Source: three-view drawing plus pictorial views. Frame: mm from the lowest corner of the part. A direction names the side the tool comes from. Give positions to 0.01 mm unless a question says otherwise; leave off trailing zeros. Loops run counter-clockwise (first coordinate to the right, second up) from the corner with the lowest first, then second, coordinate; pieces in that order, holes last. Notation, with made-up numbers: (-37, -9) -> (-24, -9) arc R37 cw to (-24, 29) -> close; hole circle Ø2 at (16, 61). An arc over 180 degrees is marked (long way). Answer as a JSON object with one key per item and string values. Group by question number.
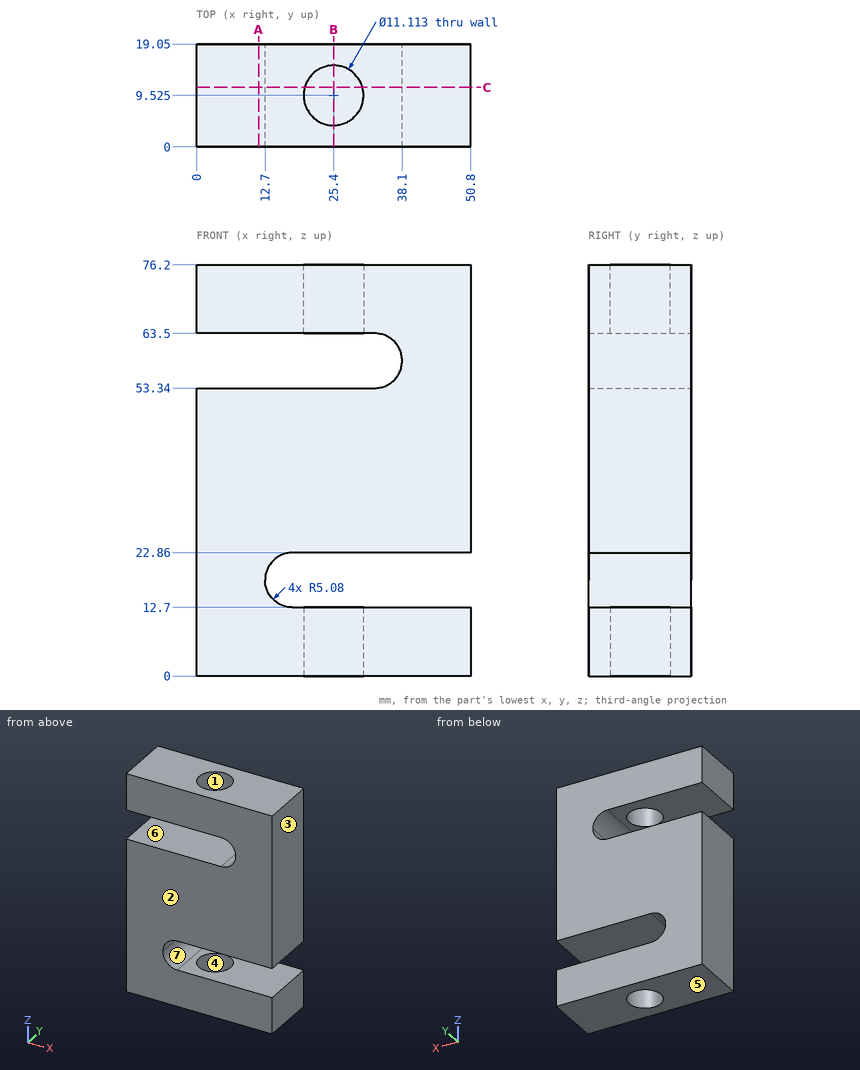
(1) Section query B-B on x = 25.4. Return the cut outline in (y, z).
(2) Section query C-C on y = 11. State how many separate pieces and enclosed holes the cut face has, plus the area to 3 significant figures.
(3) Access query for the marked faces 4, 5, 6 and 7. Directions: +Z, -Z, +X, -X, +Y, -Y. A direction counts if a zero-diameter tool reaches every point of the face in a straight line with its end or side. Return the directions, or none.
(4) First-contact query: pin 1 (6 mm diameter, centred on x = 24, y = 4.5, fed in from -Z); pin 2 (9 mm diameter, centred on x = 25.4, y = 9.525, fed in from -Z); pin 3 (4 mm diameter, centred on y = 5, z = 18, fed in from +X). Flat tips, straight axial feed; report the tip coordinate or a pass-through.
(5) Mould query, pull axis X, two halves, no side actions, for the marked faces 1, 2 and 3. Classes: pulls with the +X half, pulls with the -X half, needs draft (parallel to the pull), parting line crosses it, or undercut.
(6) Section query A-A on x = 11.5. Return the cut outline in (y, z), plus the area to 3 significant figures.
(7) Material intervals for line 1 (Z direction, x = 30.5, y = 2.5); line 2 (Y direction, x = 25.4, z = 67); line 3 (Z direction, x = 46.5, y = 2.75), sorted ascending. Write a range as from..to.
Result:
{
 "1": {"outline": "(0, 0) -> (3.97, 0) -> (3.97, 12.7) -> (0, 12.7) -> close; (0, 22.86) -> (19.05, 22.86) -> (19.05, 53.34) -> (0, 53.34) -> close; (0, 63.5) -> (3.97, 63.5) -> (3.97, 76.2) -> (0, 76.2) -> close; (15.08, 0) -> (19.05, 0) -> (19.05, 12.7) -> (15.08, 12.7) -> close; (15.08, 63.5) -> (19.05, 63.5) -> (19.05, 76.2) -> (15.08, 76.2) -> close"},
 "2": {"separate pieces": "3", "enclosed holes": "0", "area": "2,850 mm²"},
 "3": {"face 4": "-Z", "face 5": "-Z, +X, -X, +Y, -Y", "face 6": "-X, +Y, -Y", "face 7": "+X, +Y, -Y"},
 "4": {"pin 1": "z = 0", "pin 2": "z = 22.86", "pin 3": "x = 13.21"},
 "5": {"face 1": "undercut", "face 2": "needs draft", "face 3": "pulls with the +X half"},
 "6": {"outline": "(0, 0) -> (19.05, 0) -> (19.05, 53.34) -> (0, 53.34) -> close; (0, 63.5) -> (19.05, 63.5) -> (19.05, 76.2) -> (0, 76.2) -> close", "area": "1,260 mm²"},
 "7": {"line 1": "0..12.7, 22.86..53.34, 63.5..76.2", "line 2": "0..3.97, 15.08..19.05", "line 3": "0..12.7, 22.86..76.2"}
}
